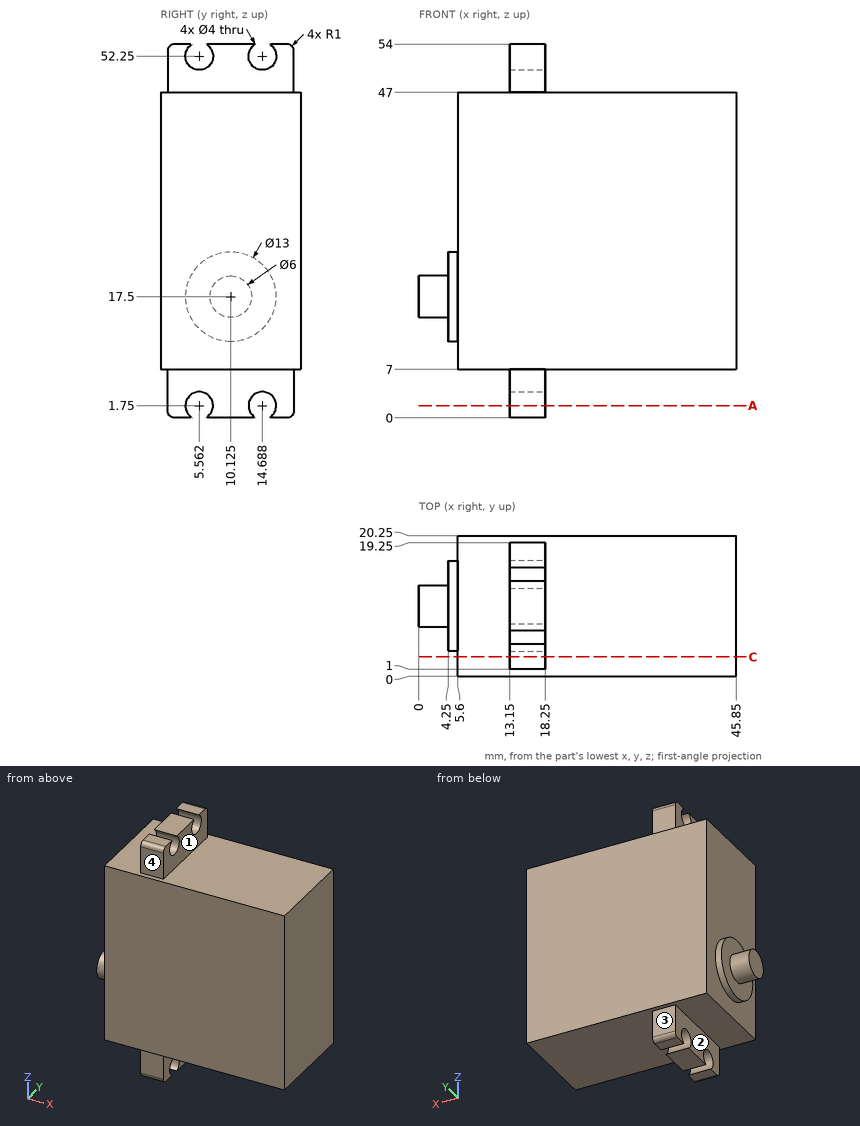
Geometry: see drawing. Coordinates: mm, zero at the bounding-box minimum. A direction names the side the tool comes from. Give positions to 0.01 mm unless a question says otherwise; leave off trailing zeros. Order: outer loops, then holes, each group sorted by start corner. A loop starts at its lowest first (then second) coordinate and runs counter-clockwise, first axis right, second up.
1. Cut plane C-C (y = 2.75). Return loops of the section in (x, z), and give its area (3 significant figures).
Computed:
outline: (5.6, 7) - (13.15, 7) - (13.15, 0) - (18.25, 0) - (18.25, 7) - (45.85, 7) - (45.85, 47) - (18.25, 47) - (18.25, 54) - (13.15, 54) - (13.15, 47) - (5.6, 47) - close
area: 1,680 mm2
2. Set-up query: the marked faces 1, 2, 3 and 4. Return all of +Z, -Z, +X, -X, +Y, -Y with unobstructed straight access to the full face (end or side cutting, diameter ignored); none if empty.
Computed:
face 1: +Z, +X, +Y, -Y
face 2: -Z, -X, +Y, -Y
face 3: -Z, +X, -X, +Y
face 4: +Z, +X, -X, -Y
3. Cut plane A-A (z = 1.75). Return loops of the section in (x, y).
Computed:
outline: (13.15, 1) - (18.25, 1) - (18.25, 3.56) - (13.15, 3.56) - close; (13.15, 7.56) - (18.25, 7.56) - (18.25, 12.69) - (13.15, 12.69) - close; (13.15, 16.69) - (18.25, 16.69) - (18.25, 19.25) - (13.15, 19.25) - close
4. Pin query (flat end, axial travel): pin 1 Ø3.5 at (y, z) = (10, 2) entering from +X; pin 2 Ø3.5 at (y, z) = (13, 5) entering from -X; pin 3 Ø6 at (x, y) = (33, 10.5) entering from +Z. Return the tip coordinate at first contact, or that it passes through.
Computed:
pin 1: stops at x = 18.25
pin 2: stops at x = 13.15
pin 3: stops at z = 47
5. Line query: probe 1 along Y at (x, z) = (14.4, 52.25); probe 2 along X at (y, z) = (10.5, 21); probe 3 along Z at (x, y) = (22, 18.25). Output: solid intervals per line, ascending.
Computed:
probe 1: y = 1 to 3.56, 7.56 to 12.69, 16.69 to 19.25
probe 2: x = 4.25 to 45.85
probe 3: z = 7 to 47
